Can you work these out from the model? Positions are in its coordinate system, mm. A direction names the side the tool comes from. Round coordinates to 2 decimals unless told otherwise and drop trailing zeros. Order: outer loops, then holes, each group sorted by start corner. A loop starts at its lowest first (then second) coordinate and runs counter-clockwise, first axis right, second up. Notation, with made-up numbers: (62, -12.75) -> (70, -12.75) arc R15 ccw to (70, 12.25) -> close; hole circle Ø3 at (18, 26.5). An arc over 180 degrees is marked (long way). Use a Markdown table: item, result. Add a question column.
Q1. I need wall thicknesses on line 1 along Z through (x, y) = (38.1, 0.9); line 2 along Y through (x, z) = (30, -710.5). Which ranges of each line are inside material? Lowest first, please. Write a range as [from, to].
Q2. We'd pull the mould along Y, two halves only. Please class faces 1 (the face through (27, 2.286, -703)), 2 (the face through (1.127, 37.831, -734.548)), 3 (the face through (25.131, 1.127, -725.952)): +Y half, -Y half, draft (parallel to the pull), parting line (faces both ways), or undercut.
Q3. If we section it at B-B on x = 12.7: List the corners of the cut face in (y, z) for me.
Q4. I'm going to push flat-ended pins straight in: pin 1 Ø3 at (x, z) = (30, -694.5) entering from +Y; pin 2 Ø5 at (y, z) = (25.4, -698.5) entering from +X; pin 3 Ø3.5 at (y, z) = (38.1, -736.6) entering from -X. Where does each tip first touch, or does it pass through?
Q5. If we section it at A-A on z = -698.5: List the corners of the cut face in (x, y) for me, plus the area to 3 significant figures.
Q6. For faces 4 (the face through (2.286, 27, -703)), 5 (the face through (1.13, 37.65, -687.82)), which set-ups out of +Z, -Z, +X, -X, +Y, -Y let a thin tool reach every point of the face, with its end or its side?
```python
from build123d import *

# Parameters (mm, degrees)
CUT_EXTRUDE1_START       = 14.7701
CUT_EXTRUDE1_OUTLINE_W   = 2.286
CUT_EXTRUDE1_OUTLINE_H   = 127
CUT_EXTRUDE1_DEPTH       = 8.5598
CUT_EXTRUDE1_START_2     = 27.4701
CUT_EXTRUDE1_2_OUTLINE_W = 2.286
CUT_EXTRUDE1_2_OUTLINE_H = 127
CUT_EXTRUDE1_2_DEPTH     = 8.5598
CUT_EXTRUDE1_START_3     = 40.1701
CUT_EXTRUDE1_3_OUTLINE_W = 2.286
CUT_EXTRUDE1_3_OUTLINE_H = 127
CUT_EXTRUDE1_3_DEPTH     = 8.4709
CUT_EXTRUDE1_START_4     = 2.286
CUT_EXTRUDE1_4_OUTLINE_W = 2.286
CUT_EXTRUDE1_4_OUTLINE_H = 127
CUT_EXTRUDE1_4_DEPTH     = 8.3439
CUT_EXTRUDE1_5_OUTLINE_R = 2.0701
CUT_EXTRUDE1_5_DEPTH     = 3.0988
CUT_EXTRUDE1_START_5     = 10.6299
CUT_EXTRUDE1_6_OUTLINE_W = 2.286
CUT_EXTRUDE1_6_OUTLINE_H = 127
CUT_EXTRUDE1_6_DEPTH     = 40.1701
CUT_EXTRUDE1_START_6     = -1
CUT_EXTRUDE1_7_OUTLINE_R = 2.0701
CUT_EXTRUDE1_7_DEPTH     = 3.286
CUT_EXTRUDE1_START_7     = -749.3
CUT_EXTRUDE1_8_DEPTH     = 127
CUT_EXTRUDE1_START_8     = 564.229492087
CUT_EXTRUDE1_9_OUTLINE_W = 3.286
CUT_EXTRUDE1_9_OUTLINE_H = 75
CUT_EXTRUDE1_9_DEPTH     = 2.770507913
CHAMFER1_SIZE            = 2.159
BOSS_EXTRUDE1_START      = -2.286
BOSS_EXTRUDE1_DEPTH      = 2.286
BOSS_EXTRUDE2_START      = -2.286
BOSS_EXTRUDE2_DEPTH      = 2.286
SKETCH4_W                = 50.8
SKETCH4_H                = 50.8
CUT_EXTRUDE2_DEPTH       = 36.181674144
BOSS_EXTRUDE3_DEPTH      = 2.286
BOSS_EXTRUDE4_START      = -2.286
BOSS_EXTRUDE4_DEPTH      = 2.286
CHAMFER2_SIZE            = 2.159


with BuildPart() as part:
    # Cut-Extrude1: read off the stored shape, not the designer's step
    # Cut-Extrude1 outline → Cut-Extrude1 (new body)
    with BuildSketch(Plane(origin=(0, 0, 0), x_dir=(1, 0, 0), z_dir=(0, 1, 0)).offset(CUT_EXTRUDE1_START)):
        with Locations((1.143, 685.8)):
            Rectangle(CUT_EXTRUDE1_OUTLINE_W, CUT_EXTRUDE1_OUTLINE_H)
    extrude(amount=CUT_EXTRUDE1_DEPTH)



with BuildPart() as body_2:
    # Cut-Extrude1 2 outline → Cut-Extrude1 2 (new body)
    with BuildSketch(Plane(origin=(0, 0, 0), x_dir=(1, 0, 0), z_dir=(0, 1, 0)).offset(CUT_EXTRUDE1_START_2)):
        with Locations((1.143, 685.8)):
            Rectangle(CUT_EXTRUDE1_2_OUTLINE_W, CUT_EXTRUDE1_2_OUTLINE_H)
    extrude(amount=CUT_EXTRUDE1_2_DEPTH)


with BuildPart() as body_3:
    # Cut-Extrude1 3 outline → Cut-Extrude1 3 (new body)
    with BuildSketch(Plane(origin=(0, 0, 0), x_dir=(1, 0, 0), z_dir=(0, 1, 0)).offset(CUT_EXTRUDE1_START_3)):
        with Locations((1.143, 685.8)):
            Rectangle(CUT_EXTRUDE1_3_OUTLINE_W, CUT_EXTRUDE1_3_OUTLINE_H)
    extrude(amount=CUT_EXTRUDE1_3_DEPTH)


with BuildPart() as body_4:
    # Cut-Extrude1 4 outline → Cut-Extrude1 4 (new body)
    with BuildSketch(Plane(origin=(0, 0, 0), x_dir=(1, 0, 0), z_dir=(0, 1, 0)).offset(CUT_EXTRUDE1_START_4)):
        with Locations((1.143, 685.8)):
            Rectangle(CUT_EXTRUDE1_4_OUTLINE_W, CUT_EXTRUDE1_4_OUTLINE_H)
    extrude(amount=CUT_EXTRUDE1_4_DEPTH)

    # Cut-Extrude1 5 outline → Cut-Extrude1 5 (add)
    with BuildSketch(Plane(origin=(0, 0, 0), x_dir=(1, 0, 0), z_dir=(0, 1, 0))):
        with BuildLine():
            ThreePointArc((23.3299, 622.3), (23.936218252, 623.763781748), (25.4, 624.3701))
            ThreePointArc((25.4, 624.3701), (26.863781748, 623.763781748), (27.4701, 622.3))
            Line((27.4701, 622.3), (50.8, 622.3))
            Line((50.8, 622.3), (50.8, 747.141))
            Line((50.8, 747.141), (48.641, 749.3))
            Line((48.641, 749.3), (0, 749.3))
            Line((0, 749.3), (0, 622.3))
            Line((0, 622.3), (23.3299, 622.3))
        make_face()
        with Locations((12.7, 635)):
            Circle(CUT_EXTRUDE1_5_OUTLINE_R, mode=Mode.SUBTRACT)
        with Locations((25.4, 647.7)):
            Circle(CUT_EXTRUDE1_5_OUTLINE_R, mode=Mode.SUBTRACT)
        with Locations((12.7, 660.4)):
            Circle(CUT_EXTRUDE1_5_OUTLINE_R, mode=Mode.SUBTRACT)
        with Locations((25.4, 673.1)):
            Circle(CUT_EXTRUDE1_5_OUTLINE_R, mode=Mode.SUBTRACT)
        with Locations((38.1, 635)):
            Circle(CUT_EXTRUDE1_5_OUTLINE_R, mode=Mode.SUBTRACT)
        with Locations((38.1, 660.4)):
            Circle(CUT_EXTRUDE1_5_OUTLINE_R, mode=Mode.SUBTRACT)
        with Locations((12.7, 685.8)):
            Circle(CUT_EXTRUDE1_5_OUTLINE_R, mode=Mode.SUBTRACT)
        with Locations((12.7, 711.2)):
            Circle(CUT_EXTRUDE1_5_OUTLINE_R, mode=Mode.SUBTRACT)
        with Locations((25.4, 698.5)):
            Circle(CUT_EXTRUDE1_5_OUTLINE_R, mode=Mode.SUBTRACT)
        with Locations((12.7, 736.6)):
            Circle(CUT_EXTRUDE1_5_OUTLINE_R, mode=Mode.SUBTRACT)
        with Locations((25.4, 723.9)):
            Circle(CUT_EXTRUDE1_5_OUTLINE_R, mode=Mode.SUBTRACT)
        with Locations((38.1, 685.8)):
            Circle(CUT_EXTRUDE1_5_OUTLINE_R, mode=Mode.SUBTRACT)
        with Locations((38.1, 711.2)):
            Circle(CUT_EXTRUDE1_5_OUTLINE_R, mode=Mode.SUBTRACT)
        with Locations((38.1, 736.6)):
            Circle(CUT_EXTRUDE1_5_OUTLINE_R, mode=Mode.SUBTRACT)
    extrude(amount=CUT_EXTRUDE1_5_DEPTH)


with BuildPart() as part_1:
    add(part.part)

    add(body_2.part)  # Cut-Extrude1 6 merges body 2

    add(body_3.part)  # Cut-Extrude1 6 merges body 3

    add(body_4.part)  # Cut-Extrude1 6 merges body 4
    # Cut-Extrude1 6 outline → Cut-Extrude1 6 (add)
    with BuildSketch(Plane(origin=(0, 0, 0), x_dir=(1, 0, 0), z_dir=(0, 1, 0)).offset(CUT_EXTRUDE1_START_5)):
        with Locations((1.143, 685.8)):
            Rectangle(CUT_EXTRUDE1_6_OUTLINE_W, CUT_EXTRUDE1_6_OUTLINE_H)
    extrude(amount=CUT_EXTRUDE1_6_DEPTH)

    # Cut-Extrude1 7 outline → Cut-Extrude1 7 (cut)
    with BuildSketch(Plane.YZ.offset(CUT_EXTRUDE1_START_6)):
        with BuildLine():
            ThreePointArc((23.3299, -622.3), (23.936218252, -623.763781748), (25.4, -624.3701))
            ThreePointArc((25.4, -624.3701), (26.863781748, -623.763781748), (27.4701, -622.3))
            Line((27.4701, -622.3), (23.3299, -622.3))
        make_face()
        with Locations((25.4, -723.9)):
            Circle(CUT_EXTRUDE1_7_OUTLINE_R)
        with Locations((25.4, -698.5)):
            Circle(CUT_EXTRUDE1_7_OUTLINE_R)
        with Locations((25.4, -673.1)):
            Circle(CUT_EXTRUDE1_7_OUTLINE_R)
        with Locations((25.4, -647.7)):
            Circle(CUT_EXTRUDE1_7_OUTLINE_R)
        with Locations((12.7, -736.6)):
            Circle(CUT_EXTRUDE1_7_OUTLINE_R)
        with Locations((12.7, -711.2)):
            Circle(CUT_EXTRUDE1_7_OUTLINE_R)
        with Locations((12.7, -685.8)):
            Circle(CUT_EXTRUDE1_7_OUTLINE_R)
        with Locations((12.7, -660.4)):
            Circle(CUT_EXTRUDE1_7_OUTLINE_R)
        with Locations((12.7, -635)):
            Circle(CUT_EXTRUDE1_7_OUTLINE_R)
        with Locations((38.1, -736.6)):
            Circle(CUT_EXTRUDE1_7_OUTLINE_R)
        with Locations((38.1, -711.2)):
            Circle(CUT_EXTRUDE1_7_OUTLINE_R)
        with Locations((38.1, -685.8)):
            Circle(CUT_EXTRUDE1_7_OUTLINE_R)
        with Locations((38.1, -660.4)):
            Circle(CUT_EXTRUDE1_7_OUTLINE_R)
        with Locations((38.1, -635)):
            Circle(CUT_EXTRUDE1_7_OUTLINE_R)
    extrude(amount=CUT_EXTRUDE1_7_DEPTH, mode=Mode.SUBTRACT)

    # Cut-Extrude1 8 outline → Cut-Extrude1 8 (cut)
    with BuildSketch(Plane.XY.offset(CUT_EXTRUDE1_START_7)):
        with BuildLine():
            ThreePointArc((3.0988, 0), (0.907617506, 0.907617506), (0, 3.0988))
            Line((0, 3.0988), (2.4e-08, 50))
            Line((2.4e-08, 50), (-1, 50))
            Line((-1, 50), (-1, -1))
            Line((-1, -1), (50.8, -1))
            Line((50.8, -1), (50.8, 0))
            Line((50.8, 0), (3.0988, 0))
        make_face()
        with BuildLine():
            Line((3.0988, 2.286), (50.8, 2.286))
            Line((50.8, 2.286), (50.8, 3.0988))
            Line((50.8, 3.0988), (2.286, 3.0988))
            ThreePointArc((2.286, 3.0988), (2.524063608, 2.524063608), (3.0988, 2.286))
        make_face()
    extrude(amount=CUT_EXTRUDE1_8_DEPTH, mode=Mode.SUBTRACT)

    # Cut-Extrude1 9 outline → Cut-Extrude1 9 (cut)
    with BuildSketch(Plane(origin=(0, 0, 0), x_dir=(1, 0, 0), z_dir=(0, 0.7071067811865511, -0.7071067811865441)).offset(CUT_EXTRUDE1_START_8)):
        with Locations((0.643, 459.5)):
            Rectangle(CUT_EXTRUDE1_9_OUTLINE_W, CUT_EXTRUDE1_9_OUTLINE_H)
    extrude(amount=CUT_EXTRUDE1_9_DEPTH, mode=Mode.SUBTRACT)

    # Chamfer1
    chamfer1_edges = [part_1.edges().sort_by_distance(p)[0] for p in [
        (1.143, 50.8, -622.3),
        (50.8, 1.143, -622.3),
    ]]
    chamfer(chamfer1_edges, length=CHAMFER1_SIZE)

    # Sketch2 → Boss-Extrude1 (add)
    with BuildSketch(Plane(origin=(2.286, 0, 0), x_dir=(0, 0, -1), z_dir=(1, 0, 0)).offset(BOSS_EXTRUDE1_START)):
        with BuildLine():
            Line((622.3, 27.4701), (622.3, 23.3299))
            ThreePointArc((622.3, 23.3299), (624.3701, 25.4), (622.3, 27.4701))
        make_face()
    extrude(amount=BOSS_EXTRUDE1_DEPTH)

    # Sketch3 → Boss-Extrude2 (add)
    with BuildSketch(Plane(origin=(0, 2.286, 0), x_dir=(1, 0, 0), z_dir=(0, 1, 0)).offset(BOSS_EXTRUDE2_START)):
        with BuildLine():
            Line((23.3299, 622.3), (27.4701, 622.3))
            ThreePointArc((27.4701, 622.3), (25.4, 624.3701), (23.3299, 622.3))
        make_face()
    extrude(amount=BOSS_EXTRUDE2_DEPTH)

    # Sketch4 → Cut-Extrude2 (cut)
    with BuildSketch(Plane.XY.offset(-622.3)):
        with Locations((25.4, 25.4)):
            Rectangle(SKETCH4_W, SKETCH4_H)
    extrude(amount=-CUT_EXTRUDE2_DEPTH, mode=Mode.SUBTRACT)

    # Sketch5 → Boss-Extrude3 (add)
    with BuildSketch(Plane.XZ):
        with BuildLine():
            Line((38.878035938, -658.481674144), (37.321964062, -658.481674144))
            ThreePointArc((37.321964062, -658.481674144), (38.1, -662.4701), (38.878035938, -658.481674144))
        make_face()
        with BuildLine():
            Line((13.478035938, -658.481674144), (11.921964062, -658.481674144))
            ThreePointArc((11.921964062, -658.481674144), (12.7, -662.4701), (13.478035938, -658.481674144))
        make_face()
    extrude(amount=-BOSS_EXTRUDE3_DEPTH)

    # Sketch6 → Boss-Extrude4 (add)
    with BuildSketch(Plane(origin=(2.286, 0, 0), x_dir=(0, 0, -1), z_dir=(1, 0, 0)).offset(BOSS_EXTRUDE4_START)):
        with BuildLine():
            Line((658.481674144, 38.878035938), (658.481674144, 37.321964062))
            ThreePointArc((658.481674144, 37.321964062), (662.4701, 38.1), (658.481674144, 38.878035938))
        make_face()
        with BuildLine():
            Line((658.481674144, 11.921964062), (658.481674144, 13.478035938))
            ThreePointArc((658.481674144, 13.478035938), (662.4701, 12.7), (658.481674144, 11.921964062))
        make_face()
    extrude(amount=BOSS_EXTRUDE4_DEPTH)

    # Chamfer2
    chamfer2_edges = [part_1.edges().sort_by_distance(p)[0] for p in [
        (50.8, 1.143, -658.481674144),
        (1.143, 50.8, -658.481674144),
    ]]
    chamfer(chamfer2_edges, length=CHAMFER2_SIZE)


solid = part_1.part
```
Answer below:
| question | item | result |
|---|---|---|
| 1 | line 1 | [-749.3, -738.67], [-734.53, -713.27], [-709.13, -687.87], [-683.73, -658.48] |
| 1 | line 2 | [0, 2.29] |
| 2 | face 1 | +Y half |
| 2 | face 2 | undercut |
| 2 | face 3 | draft |
| 3 | outline | (0, -749.3) -> (2.29, -749.3) -> (2.29, -738.67) -> (0, -738.67) -> close; (0, -734.53) -> (2.29, -734.53) -> (2.29, -713.27) -> (0, -713.27) -> close; (0, -709.13) -> (2.29, -709.13) -> (2.29, -687.87) -> (0, -687.87) -> close; (0, -683.73) -> (2.29, -683.73) -> (2.29, -658.48) -> (0, -658.48) -> close |
| 4 | pin 1 | y = 2.29 |
| 4 | pin 2 | x = 2.29 |
| 4 | pin 3 | through |
| 5 | outline | (0, 3.1) arc R3.1 ccw to (3.1, 0) -> (23.33, 0) -> (23.33, 2.29) -> (3.1, 2.29) arc R0.81 cw to (2.29, 3.1) -> (2.29, 23.33) -> (0, 23.33) -> close; (0, 27.47) -> (2.29, 27.47) -> (2.29, 50.8) -> (0, 50.8) -> close; (27.47, 0) -> (50.8, 0) -> (50.8, 2.29) -> (27.47, 2.29) -> close |
| 5 | area | 206 mm² |
| 6 | face 4 | +Z, -Z, +X, +Y |
| 6 | face 5 | +X, -X |
